Input: part model. Units: mm. Frame: model coordinates. A direction names the side the tool comes from. Round coordinates to 2 decimals unless told otherwise and drop trailing zeros. Order: outer loops, then holes, each group sorted by start corner. A loop starts at its lowest first (then second) coordinate and runs counter-clockwise, first axis right, second up. Notation, with made-up numbers: M 17.5,82 L 71.5,82 A17 ccw 71.5,91 Z; hole C -7,49 d6. An arc over 180 degrees is marked long. One line per question, with ' | ' between items.
```python
from build123d import *

# Parameters (mm, degrees)
F0_R     = 3
F1_DEPTH = 1.8
F2_R     = 1.5
F3_DEPTH = 10
F4_R     = 0.5


with BuildPart() as f1:
    # F0 (on Top) → F1 (new body)
    with BuildSketch(Plane.XY):
        with Locations((0, 0.551688)):
            Circle(F0_R)
    extrude(amount=F1_DEPTH)

    # F2 (on face) → F3 (join)
    with BuildSketch(Plane(origin=(0, 0, 0), x_dir=(1, 0, 0), z_dir=(0, 0, -1))):
        with Locations((0, -0.551688)):
            Circle(F2_R)
    extrude(amount=F3_DEPTH)

    # F4
    f4_edges = [f1.edges().sort_by_distance(p)[0] for p in [
        (-3, 0.551688, 1.8),
    ]]
    fillet(f4_edges, radius=F4_R)


solid = f1.part
```
Item 1: Access query for faces 1 (the cylindrical face through (-1.5, 0.5, -4.9)), 2 (the flat face through (0, 1, -10)). Directions: +Z, -Z, +X, -X, +Y, -Y. A direction counts if a zero-diameter tool reaches every point of the face in a straight line with its end or side. Return the directions, or none.
Report:
face 1: -Z | face 2: -Z, +X, -X, +Y, -Y
Item 2: Section query B-B, the plane z = -8.75. Return loops of the section in (x, y).
Report:
outline: C 0,0.55 d3
Item 3: Line query: line 1 along Z through (x, y) = (2.35, 0.8); line 2 along Y through (x, z) = (0.95, -7.25); line 3 along X through (y, z) = (-0.5, -6.25). Output: solid intervals per line, ascending. Write a range as from..to.
Report:
line 1: 0..1.8 | line 2: -0.61..1.71 | line 3: -1.07..1.07
Item 4: Section query A-A, the plane x = 0. Return loops of the section in (y, z), plus the area to 3 significant figures.
Report:
outline: M -2.45,0 L -0.95,0 L -0.95,-10 L 2.05,-10 L 2.05,0 L 3.55,0 L 3.55,1.3 A0.5 ccw 3.05,1.8 L -1.95,1.8 A0.5 ccw -2.45,1.3 Z | area: 40.7 mm²
Item 5: First-contact query: pin 1 (2 mm diameter, centred on y = 0, z = -3.5, fed in from +X); pin 2 (1.5 mm diameter, centred on x = 2, z = -1.5, fed in from -Y). Flat tips, straight axial feed; report the tip coordinate or a pass-through.
Report:
pin 1: x = 1.5 | pin 2: y = -0.28
